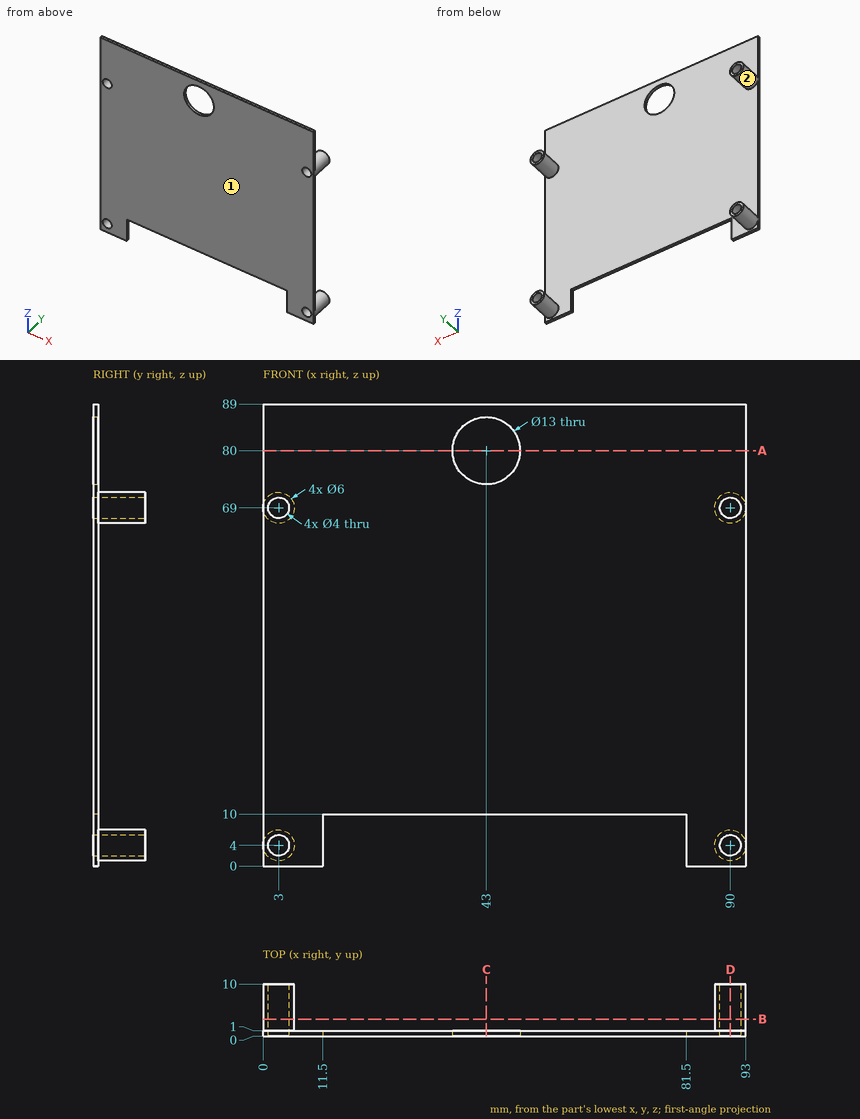
The drawing under review shows one solid part. Ordinate dimensions are in mm from its lowest x, y, z. Coordinates: 2 decimals unless noted, no trailing zeros. Write each loop counter-clockwise with the first axis right and the second up, starting at its lowest first coordinate (ties: lowest second). Pieces come first, ordered by that corner, then holes. Notation, with made-up numbers: (66, -13) - (93, -13) arc R20 cw to (93, 14) - close; hole circle Ø9 at (-22, 60.5). An arc over 180 degrees is marked (long way). Use one line per item in the form item = value.
Q1. Consider section C-C (x = 43). Write out the cut boundary in (y, z), plus the area to 3 significant figures.
Taken from the geometry:
outline = (0, 10) - (1, 10) - (1, 73.5) - (0, 73.5) - close; (0, 86.5) - (1, 86.5) - (1, 89) - (0, 89) - close
area = 66.0 mm^2
Q2. Consider section D-D (x = 90). Write out the cut boundary in (y, z), plus the area to 3 significant figures.
Taken from the geometry:
outline = (0, 0) - (1, 0) - (1, 1) - (10, 1) - (10, 2) - (0, 2) - close; (0, 6) - (10, 6) - (10, 7) - (1, 7) - (1, 66) - (10, 66) - (10, 67) - (0, 67) - close; (0, 71) - (10, 71) - (10, 72) - (1, 72) - (1, 89) - (0, 89) - close
area = 117 mm^2
Q3. Consider section A-A (z = 80). Write out the cut boundary in (x, y), plus the area to 3 significant figures.
Taken from the geometry:
outline = (0, 0) - (36.5, 0) - (36.5, 1) - (0, 1) - close; (49.5, 0) - (93, 0) - (93, 1) - (49.5, 1) - close
area = 80.0 mm^2
Q4. Insertion check: pin 1 Ø1.5 at (x, z) = (12.5, 11) entering from +Y; pin 2 Ø0.5 at (x, y) = (58, 0.5) entering from -Z. Each pin has a flat end and moves straight along its axis. Give the tip position at first contact, or say it passes through.
Taken from the geometry:
pin_1 = 1
pin_2 = 10
Q5. Consider section B-B (y = 3.25). Write out the cut boundary in (x, z).
Taken from the geometry:
outline = circle Ø6 at (3, 4); circle Ø6 at (3, 69); circle Ø6 at (90, 4); circle Ø6 at (90, 69); hole circle Ø4 at (3, 4); hole circle Ø4 at (3, 69); hole circle Ø4 at (90, 4); hole circle Ø4 at (90, 69)
Q6. The part is to be moulded in two halves that separate along Z. For the marked faces 1 and 2, say which applies: +Z half, -Z half, draft (parallel to the pull), parting line (faces both ways), or undercut.
Taken from the geometry:
face_1 = draft
face_2 = undercut
Q7. For probe 1 along X at (y, z) = (2, 69); probe 2 along Z at (x, y) = (90, 3); probe 3 along Z at (x, y) = (88.5, 8.25), list the stretches that pass through material, from the lowest coordinate up.
Taken from the geometry:
probe_1 = 0 to 1, 5 to 6, 87 to 88, 92 to 93
probe_2 = 1 to 2, 6 to 7, 66 to 67, 71 to 72
probe_3 = 1.4 to 2.68, 5.32 to 6.6, 66.4 to 67.68, 70.32 to 71.6
